Can you work these out from the model? Positions are in its coordinate system, mm. Coordinates: 2 decimals unless noted, no trailing zeros. Loops run counter-clockwise (first coordinate to the right, second up) from the corner with the lowest first, then second, coordinate; pieces in that order, holes last. Notation, with made-up numbers: M -15,-11 L 29,-11 A4 ccw 29,-5 Z; hole C 23.25,16.25 d3. An arc over 180 degrees is marked long. Answer as a JSON object with one key per item and string values. Group by question number.
Item 1: I'm going to push flat-ended pins straight in: pin 1 Ø3 at (x, y) = (3, -135.5) entering from +Z; pin 2 Ø6.5 at (x, z) = (9.5, 170.5) entering from -Y; pin 3 Ø4 at (x, z) = (7.5, 50.5) entering from -Y; pin 4 Ø1 at (x, y) = (10, -87.5) entering from -Z. Where does each tip first touch, or does it pass through?
Item 2: Suppose I cut it at B-B (x = 3). Write out the boundary of the cut face in (y, z) (3 decimals), then the cut area to 3 significant figures.
Item 3: Suppose I cut it at D-D (y = -70). Write out the boundary of the cut face in (x, z).
Item 4: Suppose I cut it at A-A (z = 52.7). Write out the boundary of the cut face in (x, y).
Item 5: If I drill on line 1 (Y direction, x = 6, z = 165); line 2 (Y direction, x = 11.5, z = 51.5); line 3 (Z direction, x = 10.25, y = -141), over which ranges is the centre line in solid material (lowest first)?
Item 6: Suppose I cut it at C-C (y = 137). Write out the boundary of the cut face in (x, z), then the cut area to 3 significant figures.
```python
from build123d import *

# Parameters (mm, degrees)
F0_R     = 19.05
F1_DEPTH = 12.7
F3_DEPTH = 12.701


# Not quite as in the source:
# - a feature names something its author has since deleted; it is built from what else it names


with BuildPart() as f1:
    # F0 (on Right) → F1 (new body)
    with BuildSketch(Plane.YZ):
        with BuildLine():
            Line((111.75, 25.4), (-177.8, 25.4))
            Line((-177.8, 25.4), (-177.8, 0))
            Line((-177.8, 0), (146.05, 0))
            Line((146.05, 0), (177.8, 0))
            Line((177.8, 0), (177.8, 25.4))
            Line((177.8, 25.4), (177.8, 228.6))
            Line((177.8, 228.6), (146.05, 228.6))
            Line((146.05, 228.6), (146.05, 107.95))
            Line((146.05, 107.95), (118.1, 80))
            Line((118.1, 80), (118.1, 31.75))
            ThreePointArc((118.1, 31.75), (116.2401280605, 27.2598719395), (111.75, 25.4))
        make_face()
        with Locations((147.9499962, 52.7)):
            Circle(F0_R, mode=Mode.SUBTRACT)
    extrude(amount=F1_DEPTH)

    # F2 (on face) → F3 (cut, through all)
    with BuildSketch(Plane.YZ.offset(12.7)):
        with BuildLine():
            ThreePointArc((166.1414, 209.55), (161.925, 213.7664), (157.7086, 209.55))
            Line((157.7086, 209.55), (157.7086, 114.3))
            ThreePointArc((157.7086, 114.3), (161.925, 110.0836), (166.1414, 114.3))
            Line((166.1414, 114.3), (166.1414, 209.55))
        make_face()
    extrude(amount=-F3_DEPTH, mode=Mode.SUBTRACT)


solid = f1.part
```
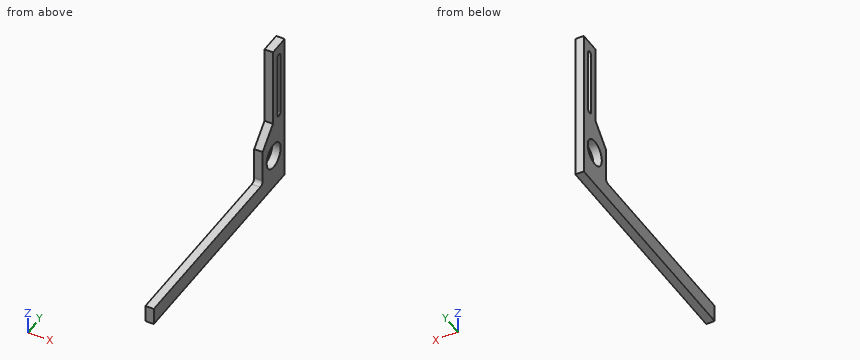
From the geometry:
{
 "1": {"pin 1": "z = 25.4", "pin 2": "y = 146.05", "pin 3": "y = 118.1", "pin 4": "z = 0"},
 "2": {"outline": "M -177.8,0 L 177.8,0 L 177.8,228.6 L 146.05,228.6 L 146.05,107.95 L 118.1,80 L 118.1,31.75 A6.35 cw 111.75,25.4 L -177.8,25.4 Z; hole C 147.95,52.7 d38.1; hole M 157.709,114.3 A4.216 ccw 166.141,114.3 L 166.141,209.55 A4.216 ccw 157.709,209.55 Z", "area": "15,400 mm2"},
 "3": {"outline": "M 0,0 L 12.7,0 L 12.7,25.4 L 0,25.4 Z"},
 "4": {"outline": "M 0,118.1 L 12.7,118.1 L 12.7,128.9 L 0,128.9 Z; M 0,167 L 12.7,167 L 12.7,177.8 L 0,177.8 Z"},
 "5": {"line 1": "146.05 to 157.71, 166.14 to 177.8", "line 2": "118.1 to 128.94, 166.96 to 177.8", "line 3": "0 to 25.4"},
 "6": {"outline": "M 0,0 L 12.7,0 L 12.7,37.11 L 0,37.11 Z; M 0,68.29 L 12.7,68.29 L 12.7,98.9 L 0,98.9 Z", "area": "860 mm2"}
}
